CAD build for the part. Positions are in the model's coordinates, mm. Face numbers are marked on the shaded views. A direction names the side the tool comes from. Give positions to 0.01 mm unless a question says otherwise; leave off trailing zeros. Order: outer loops, then holes, each group sorted by start corner. A loop starts at its lowest first (then second) coordinate and runs counter-clockwise, first axis right, second up.
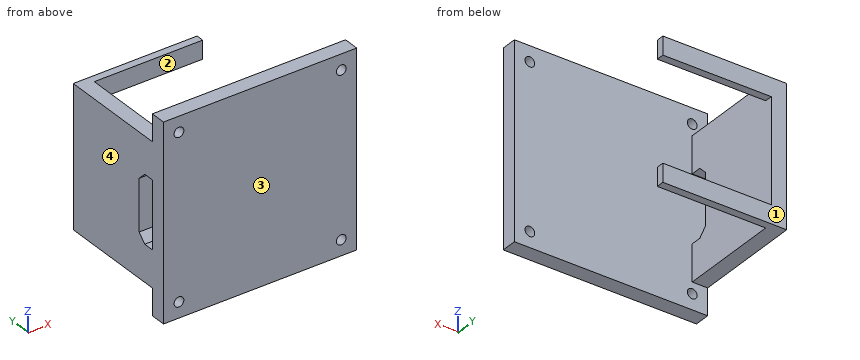
from build123d import *
from build123d.topology import SkipClean

# Parameters (mm, degrees)
SKETCH1_W           = 31.75
SKETCH1_H           = 31.75
BOSS_EXTRUDE1_DEPTH = 2.54
SKETCH3_W           = 2.54
SKETCH3_H           = 3
BOSS_EXTRUDE2_DEPTH = 18
BOSS_EXTRUDE3_DEPTH = 3.000000096
LPATTERN1_COUNT     = 2
LPATTERN1_PITCH     = 19.999999878
SKETCH7_R           = 0.8
CUT_EXTRUDE1_DEPTH  = 29.775532141
SKETCH8_W           = 2.54
SKETCH8_H           = 18
BOSS_EXTRUDE4_DEPTH = 17.000000036
SKETCH10_W          = 11
SKETCH10_H          = 3
CUT_EXTRUDE2_DEPTH  = 2.54
CHAMFER1_SIZE       = 1.27


with BuildPart() as part:
    # Sketch1 → Boss-Extrude1 (new body)
    with BuildSketch(Plane(origin=(0, 0, 0), x_dir=(1, 0, 0), z_dir=(0, 1, 0))):
        Rectangle(SKETCH1_W, SKETCH1_H)
    extrude(amount=BOSS_EXTRUDE1_DEPTH)

    # Sketch3 → Boss-Extrude2 (add)
    with BuildSketch(Plane(origin=(0, 2.54, 0), x_dir=(1, 0, 0), z_dir=(0, 1, 0))):
        with Locations((-14.605, -10.000000018)):
            Rectangle(SKETCH3_W, SKETCH3_H)
        with Locations((-14.605, 10.000000018)):
            Rectangle(SKETCH3_W, SKETCH3_H)
    extrude(amount=BOSS_EXTRUDE2_DEPTH)

    # Sketch6 → Boss-Extrude3 (add)
    with BuildSketch(Plane.XY.offset(11.500000018)):
        Polygon((-13.335, 20.54), (-13.335, 19.27), (4.479844611, 19.27), (4.482298438, 20.54), align=None)
    boss_extrude3 = extrude(amount=-BOSS_EXTRUDE3_DEPTH)

    # LPattern1: Boss-Extrude3 ×2
    with SkipClean():  # the faces are left unmerged after this step: merging them gives an invalid solid
        with Locations(*[(0, 0, -i * LPATTERN1_PITCH) for i in range(1, LPATTERN1_COUNT)]):
            add(boss_extrude3)

    # Sketch7 → Cut-Extrude1 (cut, through all)
    with SkipClean():  # the faces are left unmerged after this step: merging them gives an invalid solid
        with BuildSketch(Plane(origin=(0, 2.54, 0), x_dir=(1, 0, 0), z_dir=(0, 1, 0))):
            with Locations(Location((13.335, 13.335, 0), (0, 0, 270))):
                Circle(SKETCH7_R)
            with Locations(Location((-13.335, 13.335, 0), (0, 0, 270))):
                Circle(SKETCH7_R)
            with Locations(Location((-13.335, -13.335, 0), (0, 0, 270))):
                Circle(SKETCH7_R)
            with Locations(Location((13.335, -13.335, 0), (0, 0, 270))):
                Circle(SKETCH7_R)
        extrude(amount=-CUT_EXTRUDE1_DEPTH, mode=Mode.SUBTRACT)

    # Sketch8 → Boss-Extrude4 (add)
    with BuildSketch(Plane(origin=(0, 0, 8.500000018), x_dir=(-1, 0, 0), z_dir=(0, 0, -1))):
        with Locations((14.605, 11.54)):
            Rectangle(SKETCH8_W, SKETCH8_H)
    extrude(amount=BOSS_EXTRUDE4_DEPTH)

    # Sketch10 → Cut-Extrude2 (cut)
    with BuildSketch(Plane(origin=(-13.335, 0, 0), x_dir=(0, 0, -1), z_dir=(1, 0, 0))):
        with Locations((0, 4.04)):
            Rectangle(SKETCH10_W, SKETCH10_H)
    extrude(amount=-CUT_EXTRUDE2_DEPTH, mode=Mode.SUBTRACT)

    # Chamfer1
    chamfer1_edges = [part.edges().sort_by_distance(p)[0] for p in [
        (-14.605, 5.54, -5.5),
        (-14.605, 5.54, 5.5),
    ]]
    chamfer(chamfer1_edges, length=CHAMFER1_SIZE)


solid = part.part
1. Pin check, flat tips, straight feed: P1, Ø1.5, axis at y = 8, z = -7.5, coming from the +X side (3 decimals); P2, Ø0.9, axis at x = -15, y = 3.5, coming from the +Z side; P3, Ø1.4, axis at x = -1.5, y = 20, coming from the -Z side; P4, Ø1.5, axis at x = -7, z = 4.5, coming from the -Y side. Stop position of each tip, or through.
2. Saw through at C-C on z = 9. Give the cut face in (x, y) (3 decimals).
3. Saw through at D-D on y = 18.25. Give the cut face in (x, z) (3 decimals), plus the area to 3 significant figures.
4. Mould opens along X. For the marked faces 3 and 4 say: released by +X, released by -X, zero draft, split by the parting line, or undercut.
5. Saw through at B-B on x = -6.5. Give the cut face in (y, z) (3 decimals), plus the area to 3 significant figures.
6. Saw through at A-A on z = -3.5. Give the cut face in (x, y) (3 decimals), plus the area to 3 significant figures.
7. 3-axis set-ups, long thin cutter, end or side, ignore diameter. For the marked faces 1 and 2: which of +Z, -Z, +X, -X, +Y, -Y reach the whole face in a straight line?
8. Wall check: line 1 (Y direction, x = -5, z = -10.5); line 2 (Y direction, x = -12.5, z = 2.5); line 3 (X direction, y = 13.75, z = 10) (3 decimals). Give the ranges that are in metal, low to high.
Reported:
1. P1: stops at x = -13.335
1. P2: stops at z = 11.5
1. P3: stops at z = -11.5
1. P4: stops at y = 0
2. outline: (-15.875, 0) - (15.875, 0) - (15.875, 2.54) - (-13.335, 2.54) - (-13.335, 19.27) - (4.48, 19.27) - (4.482, 20.54) - (-15.875, 20.54) - close
3. outline: (-15.875, -11.5) - (-13.335, -11.5) - (-13.335, 11.5) - (-15.875, 11.5) - close
3. area: 58.4 mm2
4. face 3: zero draft
4. face 4: released by -X
5. outline: (0, -15.875) - (2.54, -15.875) - (2.54, 15.875) - (0, 15.875) - close; (19.27, -11.5) - (20.54, -11.5) - (20.54, -8.5) - (19.27, -8.5) - close; (19.27, 8.5) - (20.54, 8.5) - (20.54, 11.5) - (19.27, 11.5) - close
5. area: 88.3 mm2
6. outline: (-15.875, 0) - (15.875, 0) - (15.875, 2.54) - (-15.875, 2.54) - close; (-15.875, 5.54) - (-13.335, 5.54) - (-13.335, 20.54) - (-15.875, 20.54) - close
6. area: 119 mm2
7. face 1: +Z, -Z, +X, -X, +Y
7. face 2: +Z, -Z, +X
8. line 1: y = 0 to 2.54, 19.27 to 20.54
8. line 2: y = 0 to 2.54
8. line 3: x = -15.875 to -13.335
